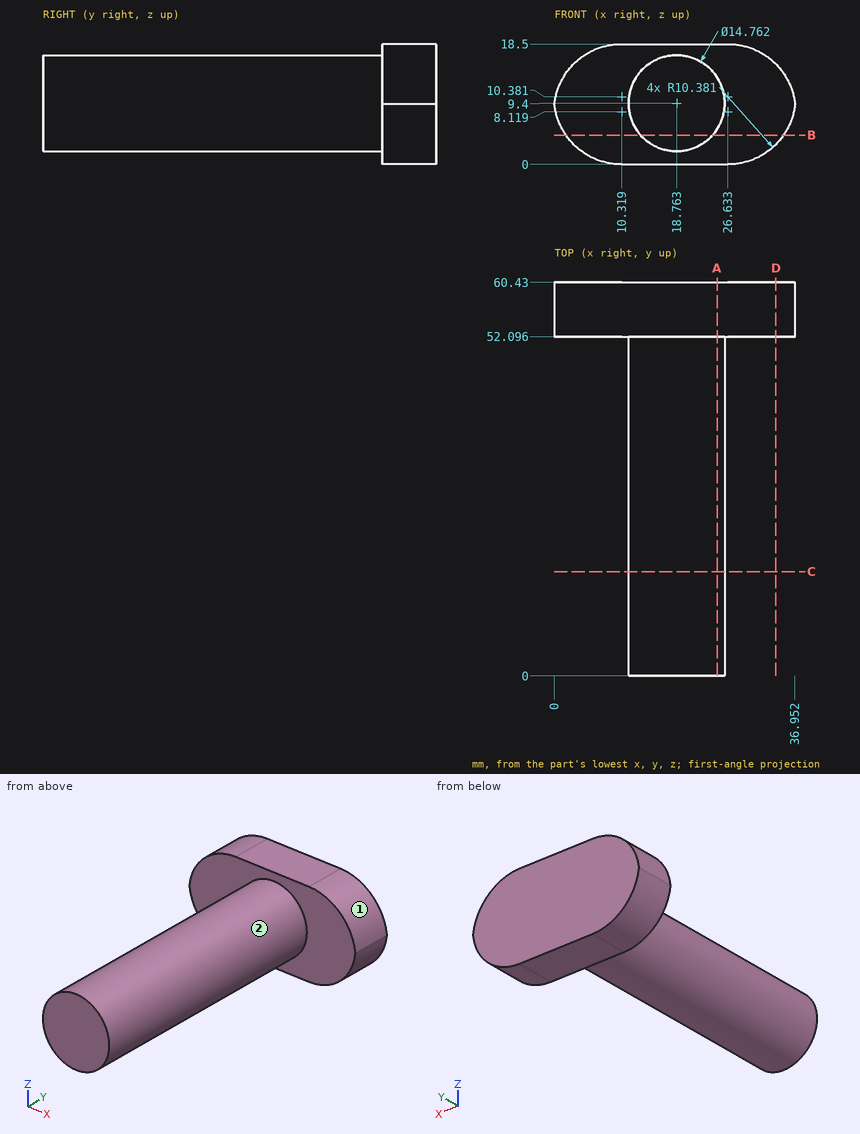
Print and shaded views of the part. All mm, measured from the part's lowest x, y and z. A direction names the side the tool comes from. Give positions to 0.01 mm unless a question says otherwise; leave off trailing zeros. Loops run counter-clockwise (first coordinate to the right, second up) from the corner with the lowest first, then second, coordinate; pieces in that order, holes last.
1) Wall check: line 1 (Y direction, x = 33.5, z = 14) (1 decimal); line 2 (X direction, y = 30, z = 9); line 3 (X direction, y = 26, z = 11.75). Give the ranges that are in metal, low to high.
2) Saw through at D-D (x = 34). Write the cut outline in (y, z) (1 decimal).
3) Saw through at B-B (z = 4.5). Write the cut outline in (x, y) (1 decimal).
4) Flat gauge pins, fed straight in: pin 1 Ø1 at (x, z) = (5, 15) entering from -Y; pin 2 Ø1 at (x, y) = (24.5, 44) entering from -Z; pin 3 Ø4 at (y, z) = (6.5, 9.5) entering from -X. Where does each tip first touch, or does it go through?
5) Tool access for the marked faces 1 and 2: list every direction of +Z, -Z, +X, -X, +Y, -Y with a clear straight run to the whole face (end or side of a thin tool).
6) Saw through at A-A (x = 25). Write the cut outline in (y, z) (1 decimal).
7) Saw through at C-C (y = 16). Write the cut outline in (x, z) (1 decimal), plus the area to 3 significant figures.
Answer block:
1. line 1: y = 52.1 to 60.4
1. line 2: x = 11.39 to 26.13
1. line 3: x = 11.77 to 25.76
2. outline: (52.1, 3.1) - (60.4, 3.1) - (60.4, 15.4) - (52.1, 15.4) - close
3. outline: (1.8, 52.1) - (13.2, 52.1) - (13.2, 0) - (24.3, 0) - (24.3, 52.1) - (35.2, 52.1) - (35.2, 60.4) - (1.8, 60.4) - close
4. pin 1: stops at y = 52.1
4. pin 2: stops at z = 4.2
4. pin 3: stops at x = 11.38
5. face 1: +Z, +X, +Y, -Y
5. face 2: -Y
6. outline: (0, 5.5) - (52.1, 5.5) - (52.1, 0) - (60.4, 0) - (60.4, 18.5) - (52.1, 18.5) - (52.1, 13.3) - (0, 13.3) - close
7. outline: circle Ø14.8 at (18.8, 9.4)
7. area: 171 mm2
